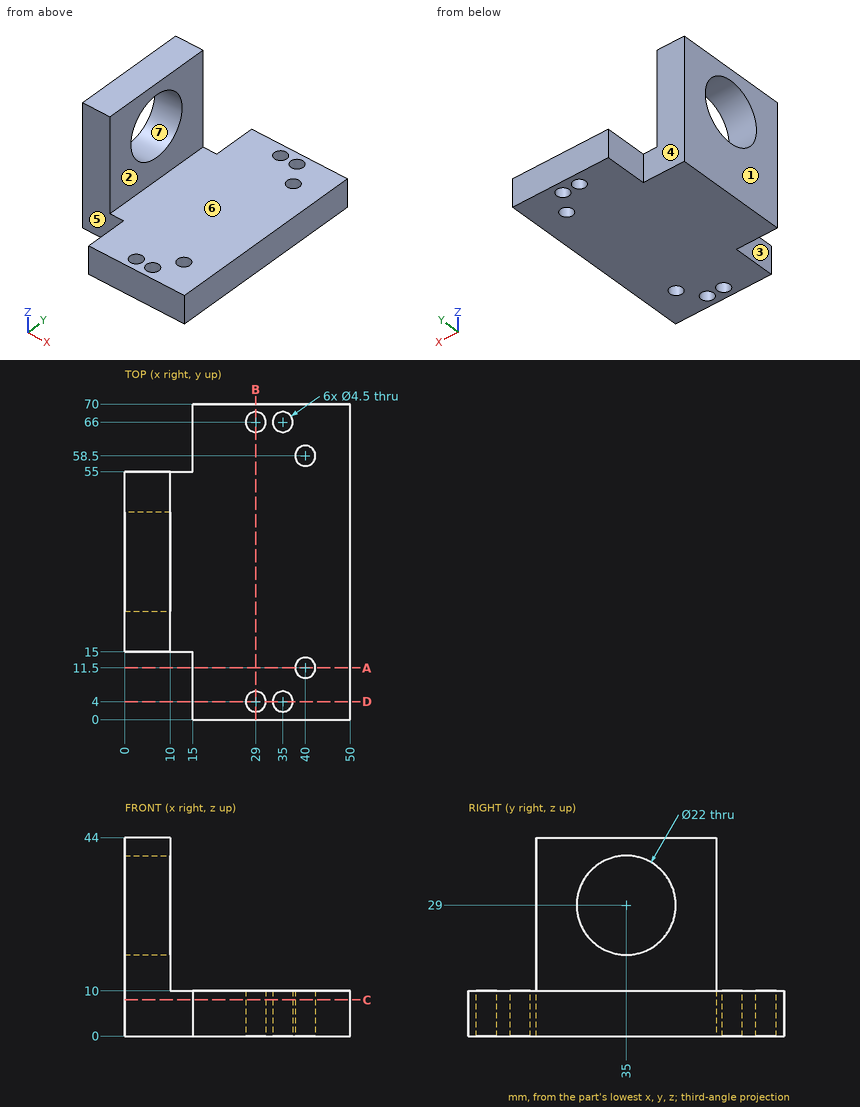
Job drawing, mm, ordinate dimensions from the low corner. One solid piece. A direction names the side the tool comes from. Give positions to 0.01 mm unless a question says otherwise; leave off trailing zeros. Loops run counter-clockwise (first coordinate to the right, second up) from the corner with the lowest first, then second, coordinate; pieces in that order, holes last. Notation, with made-up numbers: (89, 73.25) -> (103, 73.25) arc R26 cw to (103, 110.25) -> close; hole circle Ø4 at (-22, 83.25). An arc over 180 degrees is marked (long way). Write each question's results on one line, items separated by ' | '. Start each with the question number.
Q1. Pin check, flat tips, straight feed: P1, Ø2.5, axis at x = 40, y = 11.5, coming from the -Z side; P2, Ø3, axis at y = 7, z = 5.5, coming from the -X side; P3, Ø12, axis at y = 31.5, z = 24, coming from the +X side; P4, Ø12, axis at y = 19.5, z = 22, coming from the -X side. Stop position of each tip, or through.
Q2. Band-saw the part on D-D on y = 4. List the corners of the cut face in (x, z).
Q3. Band-saw the part on B-B on x = 29. List the corners of the cut face in (y, z), plus the area to 3 significant figures.
Q4. Wall check: L1, parallel to Y at x = 40, z = 2; L2, parallel to Z at x = 41, y = 25. Give the ranges that are in metal, low to high.
Q5. Pull direction Y, two halves, no side cores. Call the marked faces 5, 6 and 7: +Y half, -Y half, draft (parallel to the pull), parting line (faces both ways), or undercut.
Q6. Which spindle directions (+Z, -Z, +X, -X, +Y, -Y) get a long thin tool onto all of the face, cutting with end or side? Do the marked faces 1, 2, 3 and 4. Say none if no direction does.
Q7. Band-saw the part on C-C on z = 8. List the corners of the cut face in (x, y).
Q8. Band-saw the part on A-A on y = 11.5. List the corners of the cut face in (x, z), plus the area to 3 significant figures.
Results are:
1) P1: passes through | P2: stops at x = 15 | P3: stops at x = 10 | P4: stops at x = 0
2) outline: (15, 0) -> (26.75, 0) -> (26.75, 10) -> (15, 10) -> close; (31.25, 0) -> (32.75, 0) -> (32.75, 10) -> (31.25, 10) -> close; (37.25, 0) -> (50, 0) -> (50, 10) -> (37.25, 10) -> close
3) outline: (0, 0) -> (1.75, 0) -> (1.75, 10) -> (0, 10) -> close; (6.25, 0) -> (63.75, 0) -> (63.75, 10) -> (6.25, 10) -> close; (68.25, 0) -> (70, 0) -> (70, 10) -> (68.25, 10) -> close | area: 610 mm²
4) L1: y = 0 to 9.25, 13.75 to 56.25, 60.75 to 70 | L2: z = 0 to 10
5) face 5: -Y half | face 6: draft | face 7: undercut
6) face 1: +Z, -Z, -X, +Y, -Y | face 2: +Z, +X, +Y, -Y | face 3: +Z, -Z, -X, -Y | face 4: +Z, -Z, -X, +Y
7) outline: (0, 15) -> (15, 15) -> (15, 0) -> (50, 0) -> (50, 70) -> (15, 70) -> (15, 55) -> (0, 55) -> close; hole circle Ø4.5 at (29, 4); hole circle Ø4.5 at (29, 66); hole circle Ø4.5 at (35, 4); hole circle Ø4.5 at (35, 66); hole circle Ø4.5 at (40, 11.5); hole circle Ø4.5 at (40, 58.5)
8) outline: (15, 0) -> (37.75, 0) -> (37.75, 10) -> (15, 10) -> close; (42.25, 0) -> (50, 0) -> (50, 10) -> (42.25, 10) -> close | area: 305 mm²
